Can you work these out from the model? Positions are in its coordinate system, mm. A direction names the side the tool comes from. Give positions to 0.01 mm unless a question says otherwise; leave off trailing zeros. Loops run counter-clockwise (first coordinate to the right, second up) from the corner with the lowest first, then second, coordinate; pieces in that order, holes last. Notation, with made-up numbers: (-0.5, 16.5) - (36.5, 16.5) arc R14 ccw to (36.5, 27.5) - close; hole circle Ø4 at (68.25, 9). An arc over 180 degrees is marked (long way). Write item = value, one per line.
from build123d import *

# Parameters (mm, degrees)
BOSS_EXTRUDE1_DEPTH = 0.5
CUT_EXTRUDE1_DEPTH  = 0.5
CIRPATTERN1_COUNT   = 10
CIRPATTERN1_ANGLE   = 101.25
CUT_EXTRUDE3_START  = -0.5
CUT_EXTRUDE3_DEPTH  = 0.5
FILLET3_R           = 1


with BuildPart() as part:
    # Sketch1 → Boss-Extrude1 (new body)
    with BuildSketch(Plane.XY):
        with BuildLine():
            Line((-8.260223146, -4.3), (-10.732831081, -5.58715822))
            ThreePointArc((-10.732831081, -5.58715822), (0, -12.1), (10.732831081, -5.58715822))
            Line((10.732831081, -5.58715822), (8.260223146, -4.3))
            Line((8.260223146, -4.3), (5.774945887, -4.3))
            ThreePointArc((5.774945887, -4.3), (5.659072475, -4.451392897), (5.53923133, -4.5996648))
            Line((5.53923133, -4.5996648), (6.59, -6.419649523))
            ThreePointArc((6.59, -6.419649523), (5.831509763, -7.1157216), (5, -7.722693831))
            Line((5, -7.722693831), (5, -7.841555968))
            ThreePointArc((5, -7.841555968), (0, -9.3), (-5, -7.841555968))
            Line((-5, -7.841555968), (-5, -7.722693831))
            ThreePointArc((-5, -7.722693831), (-5.831509763, -7.1157216), (-6.59, -6.419649523))
            Line((-6.59, -6.419649523), (-5.53923133, -4.5996648))
            ThreePointArc((-5.53923133, -4.5996648), (-5.659072475, -4.451392897), (-5.774945887, -4.3))
            Line((-5.774945887, -4.3), (-8.260223146, -4.3))
        make_face()
    extrude(amount=BOSS_EXTRUDE1_DEPTH)

    # Sketch2 → Cut-Extrude1 (cut)
    with BuildSketch(Plane.XY.offset(0.5)):
        with BuildLine():
            Line((-10.617511084, -5.803314431), (-9.055174855, -6.258693914))
            ThreePointArc((-9.055174855, -6.258693914), (-8.704696722, -6.641173681), (-8.882127626, -7.128661083))
            Line((-8.882127626, -7.128661083), (-9.436602245, -7.573674013))
            ThreePointArc((-9.436602245, -7.573674013), (-10.066052286, -6.714506042), (-10.617511084, -5.803314431))
        make_face()
    cut_extrude1 = extrude(amount=-CUT_EXTRUDE1_DEPTH, mode=Mode.SUBTRACT)

    # CirPattern1: Cut-Extrude1 ×10 about axis
    cirpattern1_axis = Axis((0, 0, 0), (0, 0, 1))
    for i in range(1, CIRPATTERN1_COUNT):
        add(cut_extrude1.rotate(cirpattern1_axis, i * CIRPATTERN1_ANGLE / (CIRPATTERN1_COUNT - 1)), mode=Mode.SUBTRACT)

    # Sketch3 → Cut-Extrude3 (cut)
    with BuildSketch(Plane.XY.offset(0.5).offset(CUT_EXTRUDE3_START)):
        with BuildLine():
            Line((7.919995926, -7.488902759), (7.763179028, -9.281328104))
            ThreePointArc((7.763179028, -9.281328104), (9.430658528, -7.581073784), (10.732831081, -5.58715822))
            Line((10.732831081, -5.58715822), (9.668418082, -5.033059884))
            ThreePointArc((9.668418082, -5.033059884), (8.879519575, -6.321719079), (7.919995926, -7.488902759))
        make_face()
    extrude(amount=CUT_EXTRUDE3_DEPTH, mode=Mode.SUBTRACT)

    # Fillet3
    fillet3_edges = [part.edges().sort_by_distance(p)[0] for p in [
        (9.668418082, -5.033059884, 0.25),
    ]]
    fillet(fillet3_edges, radius=FILLET3_R)


solid = part.part
Q1. Imagine slicing it at B-B, the plane x = -8.5. Write out the boundary of the cut face in (y, z), then the cut area to 3 significant figures.
Output:
outline = (-7.83, 0) - (-4.42, 0) - (-4.42, 0.5) - (-7.83, 0.5) - close
area = 1.70 mm2
Q2. We'd pull the mould along Y, two halves only. Please class faces 4 (the flat face through (-1, -10, 0)), 5 (the cylindrical face through (5.84, -7.11, 0.25)), 6 (the cylindrical face through (8.56, -6.75, 0.25)): released by +Y, released by -Y, zero draft, split by the parting line, or undercut.
Output:
face_4 = zero draft
face_5 = undercut
face_6 = released by -Y
Q3. Which directions (+Z, -Z, +X, -X, +Y, -Y) give clear straight access to the entire face, cutting with the end or side of a thin tool? Please do faces 1 (the cylindrical face through (-5.82, -7.125, 0.246)), 2 (the flat face through (-1, -10, 0.5)), 3 (the flat face through (-0.46, -11.54, 0.25)).
Output:
face_1 = +Z, -Z
face_2 = +Z, +X, -X, +Y, -Y
face_3 = +Z, -Z, -Y
Q4. Imagine slicing it at A-A, the plane x = -2.75. Write out the boundary of the cut face in (y, z).
Output:
outline = (-11.25, 0) - (-8.88, 0) - (-8.88, 0.5) - (-11.25, 0.5) - close
Q5. For pin 1 (2 mm diameter, centred on x = -2.5, y = -7, fed in from +Z), with a flat end and sliding along its axis, tell me the tip position at first contact or that it passes through.
Output:
pin_1 = through
Q6. I need wall thicknesses on L1, parallel to X at y = -11.25, z = 0.2; L2, parallel to X at y = -6.5, z = 0.15; L3, parallel to Y at x = -5.75, z = 0.1. Which ranges of each line are inside material? Lowest first, please.
Output:
L1 = -3.55 to -2.75, -1.24 to -0.12, 0.97 to 1.92, 3.28 to 3.77
L2 = -8.76 to -6.51, 6.51 to 8.75
L3 = -10.65 to -10.48, -9.27 to -7.18, -4.96 to -4.33
